Could you check a few things on this model? Use its own coordinates, in mm. A direction names the side the tool comes from. Round coordinates to 2 decimals unless told otherwise and drop trailing zeros. Write each loop counter-clockwise with the first axis right and the second up, starting at its lowest first coordinate (ties: lowest second). Pieces come first, ordered by that corner, then holes. Notation, with made-up numbers: (-26, -9) -> (-10, -9) arc R9 ccw to (-10, 4) -> close; hole circle Ø8 at (-37.5, 6.25). An arc over 180 degrees is marked (long way). Answer in a Markdown table with one row per item.
from build123d import *

# Parameters (mm, degrees)
CROQUIS1_W              = 15
CROQUIS1_H              = 44
CROQUIS1_R              = 1.5
SALIENTE_EXTRUIR1_DEPTH = 5
CROQUIS2_W              = 15
CROQUIS2_H              = 5
SALIENTE_EXTRUIR2_DEPTH = 34
CROQUIS2_3_W            = 15
CROQUIS2_3_H            = 5
SALIENTE_EXTRUIR3_DEPTH = 31
CORTAR_EXTRUIR1_REACH   = 61.273
CROQUIS3_R              = 1.5
CORTAR_EXTRUIR2_REACH   = 61.273
CROQUIS4_R              = 4
CROQUIS5_W              = 6
CROQUIS5_H              = 5.854248689
CORTAR_EXTRUIR3_DEPTH   = 2
CORTAR_EXTRUIR4_DEPTH   = 3


with BuildPart() as part:
    # Croquis1 → Saliente-Extruir1 (new body)
    with BuildSketch(Plane(origin=(0, 0, 0), x_dir=(1, 0, 0), z_dir=(0, 1, 0))):
        Rectangle(CROQUIS1_W, CROQUIS1_H)
        with Locations(Location((3.5, 0, 0), (0, 0, 270))):
            Circle(CROQUIS1_R, mode=Mode.SUBTRACT)
        with Locations(Location((-3.5, 0, 0), (0, 0, 270))):
            Circle(CROQUIS1_R, mode=Mode.SUBTRACT)
    extrude(amount=-SALIENTE_EXTRUIR1_DEPTH)

    # Croquis2 → Saliente-Extruir2 (add)
    with BuildSketch(Plane.XZ.offset(5)):
        with Locations((0, -19.5)):
            Rectangle(CROQUIS2_W, CROQUIS2_H)
    extrude(amount=SALIENTE_EXTRUIR2_DEPTH)

    # Croquis2_3 → Saliente-Extruir3 (add)
    with BuildSketch(Plane.XZ.offset(5)):
        with Locations((0, 19.5)):
            Rectangle(CROQUIS2_3_W, CROQUIS2_3_H)
    extrude(amount=SALIENTE_EXTRUIR3_DEPTH)

    # Croquis3 → Cortar-Extruir1 (cut, up to next)
    with BuildSketch(Plane.XY.offset(22), mode=Mode.PRIVATE) as cortar_extruir1_sk1:
        with Locations((0, -30.5)):
            Circle(CROQUIS3_R)
    cortar_extruir1_tool1 = extrude(cortar_extruir1_sk1.sketch, amount=-CORTAR_EXTRUIR1_REACH, mode=Mode.PRIVATE) & part.part
    # Croquis3 → Cortar-Extruir1 (cut, up to next)
    with BuildSketch(Plane.XY.offset(22), mode=Mode.PRIVATE) as cortar_extruir1_sk2:
        with BuildLine():
            ThreePointArc((0, -36), (-5.303300859, -33.803300859), (-7.5, -28.5))
            Line((-7.5, -28.5), (-7.5, -36))
            Line((-7.5, -36), (0, -36))
        make_face()
    cortar_extruir1_tool2 = extrude(cortar_extruir1_sk2.sketch, amount=-CORTAR_EXTRUIR1_REACH, mode=Mode.PRIVATE) & part.part
    # Croquis3 → Cortar-Extruir1 (cut, up to next)
    with BuildSketch(Plane.XY.offset(22), mode=Mode.PRIVATE) as cortar_extruir1_sk3:
        with BuildLine():
            Line((7.5, -36), (7.5, -28.5))
            ThreePointArc((7.5, -28.5), (5.303300859, -33.803300859), (0, -36))
            Line((0, -36), (7.5, -36))
        make_face()
    cortar_extruir1_tool3 = extrude(cortar_extruir1_sk3.sketch, amount=-CORTAR_EXTRUIR1_REACH, mode=Mode.PRIVATE) & part.part
    add(cortar_extruir1_tool1.solids().sort_by_distance((0, -30.5, 22))[0], mode=Mode.SUBTRACT)
    add(cortar_extruir1_tool2.solids().sort_by_distance((-5.82474, -34.32474, 22))[0], mode=Mode.SUBTRACT)
    add(cortar_extruir1_tool3.solids().sort_by_distance((5.82474, -34.32474, 22))[0], mode=Mode.SUBTRACT)

    # Croquis4 → Cortar-Extruir2 (cut, up to next)
    with BuildSketch(Plane(origin=(0, 0, -22), x_dir=(-1, 0, 0), z_dir=(0, 0, -1)), mode=Mode.PRIVATE) as cortar_extruir2_sk1:
        with Locations((0, -30.5)):
            Circle(CROQUIS4_R)
    cortar_extruir2_tool1 = extrude(cortar_extruir2_sk1.sketch, amount=-CORTAR_EXTRUIR2_REACH, mode=Mode.PRIVATE) & part.part
    # Croquis4 → Cortar-Extruir2 (cut, up to next)
    with BuildSketch(Plane(origin=(0, 0, -22), x_dir=(-1, 0, 0), z_dir=(0, 0, -1)), mode=Mode.PRIVATE) as cortar_extruir2_sk2:
        with BuildLine():
            Line((7.5, -39), (7.5, -31.5))
            ThreePointArc((7.5, -31.5), (5.303300859, -36.803300859), (0, -39))
            Line((0, -39), (7.5, -39))
        make_face()
    cortar_extruir2_tool2 = extrude(cortar_extruir2_sk2.sketch, amount=-CORTAR_EXTRUIR2_REACH, mode=Mode.PRIVATE) & part.part
    # Croquis4 → Cortar-Extruir2 (cut, up to next)
    with BuildSketch(Plane(origin=(0, 0, -22), x_dir=(-1, 0, 0), z_dir=(0, 0, -1)), mode=Mode.PRIVATE) as cortar_extruir2_sk3:
        with BuildLine():
            ThreePointArc((0, -39), (-5.303300862, -36.803300856), (-7.5, -31.499999991))
            Line((-7.5, -31.499999991), (-7.5, -39))
            Line((-7.5, -39), (0, -39))
        make_face()
    cortar_extruir2_tool3 = extrude(cortar_extruir2_sk3.sketch, amount=-CORTAR_EXTRUIR2_REACH, mode=Mode.PRIVATE) & part.part
    add(cortar_extruir2_tool1.solids().sort_by_distance((0, -30.5, -22))[0], mode=Mode.SUBTRACT)
    add(cortar_extruir2_tool2.solids().sort_by_distance((-5.82474, -37.32474, -22))[0], mode=Mode.SUBTRACT)
    add(cortar_extruir2_tool3.solids().sort_by_distance((5.82474, -37.32474, -22))[0], mode=Mode.SUBTRACT)

    # Croquis5 → Cortar-Extruir3 (cut)
    with BuildSketch(Plane.XY.offset(-17)):
        with Locations((0, -36.072875655)):
            Rectangle(CROQUIS5_W, CROQUIS5_H)
    extrude(amount=-CORTAR_EXTRUIR3_DEPTH, mode=Mode.SUBTRACT)

    # Croquis6 → Cortar-Extruir4 (cut)
    with BuildSketch(Plane(origin=(0, 0, -22), x_dir=(-1, 0, 0), z_dir=(0, 0, -1))):
        with BuildLine():
            Line((2.125, -10.5), (-2.125, -10.5))
            Line((-2.125, -10.5), (-3.464101615, -28.5))
            ThreePointArc((-3.464101615, -28.5), (0, -26.5), (3.464101615, -28.5))
            Line((3.464101615, -28.5), (2.125, -10.5))
        make_face()
    extrude(amount=-CORTAR_EXTRUIR4_DEPTH, mode=Mode.SUBTRACT)


solid = part.part
1) Please list where these lines run through material, in increasing order: line 1 (X direction, y = -3.5, z = 0); line 2 (Z direction, x = -0.5, y = -5.5); line 3 (X direction, y = -2, z = 1).
Findings:
| item | result |
|---|---|
| line 1 | x = -7.5 to -5, -2 to 2, 5 to 7.5 |
| line 2 | z = -22 to -17, 17 to 22 |
| line 3 | x = -7.5 to -4.62, -2.38 to 2.38, 4.62 to 7.5 |
2) Imagine slicing it at A-A, the plane z = 0. Please give me the cut outline in (x, y), plus the area to 3 significant figures.
Findings:
| item | result |
|---|---|
| outline | (-7.5, -5) -> (-5, -5) -> (-5, 0) -> (-7.5, 0) -> close; (-2, -5) -> (2, -5) -> (2, 0) -> (-2, 0) -> close; (5, -5) -> (7.5, -5) -> (7.5, 0) -> (5, 0) -> close |
| area | 45.0 mm^2 |
3) For faces 1 (the face through (3, -36, -18)), 2 (the face through (7.5, -4, 0)), 3 (the face through (0, -18, 22)), 4 (the face through (0, -18, -17)), 5 (the face through (-2.8, -19.6, -20.5)), which set-ups out of +Z, -Z, +X, -X, +Y, -Y let a thin tool reach every point of the face, with its end or its side?
Findings:
| item | result |
|---|---|
| face 1 | -Y |
| face 2 | +Z, -Z, +X, +Y, -Y |
| face 3 | +Z, +X, -X, +Y, -Y |
| face 4 | +X, -X, -Y |
| face 5 | -Z |
4) Imagine slicing it at B-B, the plane y = -5.5. Please give me the cut outline in (x, z).
Findings:
| item | result |
|---|---|
| outline | (-7.5, -22) -> (7.5, -22) -> (7.5, -17) -> (-7.5, -17) -> close; (-7.5, 17) -> (7.5, 17) -> (7.5, 22) -> (-7.5, 22) -> close |
5) Imagine slicing it at C-C, the plane x = -4.5. Please give me the cut outline in (y, z).
Findings:
| item | result |
|---|---|
| outline | (-37.5, -22) -> (0, -22) -> (0, -1.12) -> (-5, -1.12) -> (-5, -17) -> (-37.5, -17) -> close; (-34.5, 17) -> (-5, 17) -> (-5, 1.12) -> (0, 1.12) -> (0, 22) -> (-34.5, 22) -> close |
6) Thinking about a two-plate mould opening in X: for faces 6 (the face through (-7.5, -4, 0)), 7 (the face through (-1.846, -34.049, -19.535)), 8 (the face through (0, -5, 0)), which applies, +X half, -X half, draft (parallel to the pull), parting line (faces both ways), or undercut?
Findings:
| item | result |
|---|---|
| face 6 | -X half |
| face 7 | undercut |
| face 8 | draft |
7) For pin 1 (2 mm diameter, centred on y = -35.5, z = -18.5, fed in from -X); pin 2 (7.5 mm diameter, centred on x = -0.5, z = 1, fed in from -Y); pin 3 (2 mm diameter, centred on y = -35, z = -18.5, fed in from +X), each with a flat end and sliding along its axis, tell me the tip position at first contact or that it passes through.
Findings:
| item | result |
|---|---|
| pin 1 | stops at x = -6.87 |
| pin 2 | stops at y = -5 |
| pin 3 | stops at x = 7.07 |
8) Imagine slicing it at D-D, the plane z = -10. Please give me the cut outline in (x, y), plus the area to 3 significant figures.
Findings:
| item | result |
|---|---|
| outline | (-7.5, -5) -> (7.5, -5) -> (7.5, 0) -> (-7.5, 0) -> close |
| area | 75.0 mm^2 |
